Part model, mm, in its own coordinate system. A direction names the side the tool comes from. Coordinates: 2 decimals unless noted, no trailing zeros. Loops run counter-clockwise (first coordinate to the right, second up) from the corner with the lowest first, then second, coordinate; pieces in that order, holes last. Notation, with made-up numbers: (37.25, -18.75) - (65.25, -18.75) arc R15 ccw to (65.25, 2.25) - close; hole circle Ø7 at (78.25, 11.5). An arc over 180 degrees is marked (long way). Use a Markdown table: item, result. Add a question column.
1) Band-saw the part on B-B (x = -183.5). Give the cut face in (y, z) (3 decimals).
2) Tool access for faces 4 (the face through (-184, 0, 178.594)), 5 (the face through (-98, 0, -162.719)), 6 (the face through (-247.904, 0, 10)): list every direction of +Z, -Z, +X, -X, +Y, -Y with a clear straight run to the whole face (end or side of a thin tool).
3) Band-saw the part on C-C (z = 256.5). Give the cut face in (x, y) (3 decimals).
4) Drop flat-ended pins along their axis: P1, Ø8, axis at y = 2, z = 206.5, coming from the -X side; P2, Ø1, axis at x = 17.5, y = 2, coming from the -Z side. Give the stop position or say it passes through.
5) Probe probe 1 along X at (y, z) = (-6, -248.5); probe 2 along Z at (x, y) = (41.5, 1); probe 3 along X at (y, z) = (6, 207). List the from-to ranges inside material, lowest first. Write a range as [from, to].
6) Band-saw the part on A-A (y = 1.75). Give the cut face in (x, z), plus the area to 3 significant figures.
7) Pull direction Z, two halves, no side cores. Call faces 1 (the face through (56.896, 0, -230)), 2 (the face through (287, 0, -296.069)), 3 (the face through (198, 0, 296.069)): +Z half, -Z half, draft (parallel to the pull), parting line (faces both ways), or undercut.
from build123d import *

# Parameters (mm, degrees)
F0_W     = 771.525
F0_H     = 296.06875
F1_DEPTH = 9.525
F2_W     = 304.8
F2_H     = 133.35
F3_DEPTH = 19.051
F4_W     = 130.175
F4_H     = 117.475
F5_DEPTH = 19.051


with BuildPart() as f1:
    # F0 (on Front) → F1 (new body, symmetric)
    with BuildSketch(Plane.XZ):
        with Locations((137.8585046741, 148.034375)):
            Rectangle(F0_W, F0_H)
        with Locations((137.8585046741, -148.034375)):
            Rectangle(F0_W, F0_H)
    extrude(amount=F1_DEPTH, both=True)

    # F2 (on face) → F3 (cut, through all)
    with BuildSketch(Plane.XZ.offset(9.525)):
        with Locations((-95.5039953259, -229.39375)):
            Rectangle(F2_W, F2_H)
    extrude(amount=-F3_DEPTH, mode=Mode.SUBTRACT)

    # F4 (on face) → F5 (cut, through all)
    with BuildSketch(Plane.XZ.offset(9.525)):
        with Locations((-182.8164953259, 237.33125)):
            Rectangle(F4_W, F4_H)
    extrude(amount=-F5_DEPTH, mode=Mode.SUBTRACT)


solid = f1.part
Answer block:
| question | item | result |
|---|---|---|
| 1 | outline | (-9.525, -162.719) - (9.525, -162.719) - (9.525, 178.594) - (-9.525, 178.594) - close |
| 2 | face 4 | +Z, -X, +Y, -Y |
| 2 | face 5 | -Z, -X, +Y, -Y |
| 2 | face 6 | +Z, -Z, -X, +Y, -Y |
| 3 | outline | (-117.729, -9.525) - (523.621, -9.525) - (523.621, 9.525) - (-117.729, 9.525) - close |
| 4 | P1 | x = -117.73 |
| 4 | P2 | z = -162.72 |
| 5 | probe 1 | [56.9, 523.62] |
| 5 | probe 2 | [-162.72, 296.07] |
| 5 | probe 3 | [-117.73, 523.62] |
| 6 | outline | (-247.9, -162.72) - (56.9, -162.72) - (56.9, -296.07) - (523.62, -296.07) - (523.62, 296.07) - (-117.73, 296.07) - (-117.73, 178.59) - (-247.9, 178.59) - close |
| 6 | area | 401,000 mm2 |
| 7 | face 1 | draft |
| 7 | face 2 | -Z half |
| 7 | face 3 | +Z half |
